from build123d import *

# Parameters (mm, degrees)
F1_DEPTH        = 5
F2_DEPTH        = 2.5
F3_R            = 8.24999
F4_R            = 13.24999
F5_R            = 13.24999
F6_R            = 15.24999
F7_DEPTH        = 4
F8_DEPTH        = 4
F9_R            = 4.99999
F11_D           = 3.1
F11_CSINK_D     = 6.1
F11_CSINK_ANGLE = 90
F13_D           = 3.1
F13_CSINK_D     = 6.1
F13_CSINK_ANGLE = 90
F14_R           = 1


# Not quite as in the source:
# - a fillet or chamfer is up to 0.001 mm smaller than in the source, because OpenCascade refuses the exact size


with BuildPart() as f1:
    # F0 (on Front) → F1 (new body, symmetric)
    with BuildSketch(Plane.XZ):
        Polygon((-20.0976822525, 0), (-7.0976822525, 0), (-7.0976822525, 8.25), (-7.0976822525, 16.5), (9.4023177475, 16.5), (9.4023177475, 0), (22.4023177475, 0), (22.4023177475, 5), (16.4023177475, 5), (14.4023177475, 5), (14.4023177475, 21.5), (-12.0976822525, 21.5), (-12.0976822525, 5), (-14.0976822525, 5), (-20.0976822525, 5), align=None)
    extrude(amount=F1_DEPTH, both=True)

    # F0 (on Front) → F2 (join, symmetric)
    with BuildSketch(Plane.XZ):
        Polygon((-14.0976822525, 23.5), (-14.0976822525, 5), (-12.0976822525, 5), (-12.0976822525, 21.5), (14.4023177475, 21.5), (14.4023177475, 5), (16.4023177475, 5), (16.4023177475, 23.5), align=None)
    extrude(amount=F2_DEPTH, both=True)

    # F3 (radius 8.25 in the source; OpenCascade refuses exactly that, so slightly less here)
    f3_edges = [f1.edges().sort_by_distance(p)[0] for p in [
        (-7.097682, 0, 16.5),
        (9.402318, 0, 16.5),
    ]]
    fillet(f3_edges, radius=F3_R)

    # F4 (radius 13.25 in the source; OpenCascade refuses exactly that, so slightly less here)
    f4_edges = [f1.edges().sort_by_distance(p)[0] for p in [
        (14.402318, -3.75, 21.5),
        (-12.097682, -3.75, 21.5),
    ]]
    fillet(f4_edges, radius=F4_R)

    # F5 (radius 13.25 in the source; OpenCascade refuses exactly that, so slightly less here)
    f5_edges = [f1.edges().sort_by_distance(p)[0] for p in [
        (14.402318, 3.75, 21.5),
        (-12.097682, 3.75, 21.5),
    ]]
    fillet(f5_edges, radius=F5_R)

    # F6 (radius 15.25 in the source; OpenCascade refuses exactly that, so slightly less here)
    f6_edges = [f1.edges().sort_by_distance(p)[0] for p in [
        (16.402318, 0, 23.5),
        (-14.097682, 0, 23.5),
    ]]
    fillet(f6_edges, radius=F6_R)

    # F7 (add): a face of the model
    f7_faces = [f1.faces().sort_by_distance(p)[0] for p in [
        (22.4023177475, 0, 2.5),
    ]]
    extrude(f7_faces, amount=F7_DEPTH)

    # F8 (add): a face of the model
    f8_faces = [f1.faces().sort_by_distance(p)[0] for p in [
        (-20.0976822525, 0, 2.5),
    ]]
    extrude(f8_faces, amount=F8_DEPTH)

    # F9 (radius 5 in the source; OpenCascade refuses exactly that, so slightly less here)
    f9_edges = [f1.edges().sort_by_distance(p)[0] for p in [
        (26.402318, -5, 2.5),
        (26.402318, 5, 2.5),
        (-24.097682, -5, 2.5),
        (-24.097682, 5, 2.5),
    ]]
    fillet(f9_edges, radius=F9_R)

    # F11 (through all)
    with Locations(Plane.XY.offset(5)):
        with Locations((-19.0976822525, 0)):
            CounterSinkHole(F11_D / 2, F11_CSINK_D / 2, counter_sink_angle=F11_CSINK_ANGLE)

    # F13 (through all)
    with Locations(Plane.XY.offset(5)):
        with Locations((21.4023177475, 0)):
            CounterSinkHole(F13_D / 2, F13_CSINK_D / 2, counter_sink_angle=F13_CSINK_ANGLE)

    # F14
    f14_edges = [f1.edges().sort_by_distance(p)[0] for p in [
        (-9.631064, -2.5, 19.033381),
        (-9.631064, 2.5, 19.033381),
        (17.902323, 5, 5),
        (-15.597687, 5, 5),
        (-12.097682, 5, 6.625005),
        (-8.21685, 5, 17.619168),
        (1.152318, 5, 21.5),
        (10.521486, 5, 17.619168),
        (14.402318, 5, 6.625005),
        (-22.633219, 3.535537, 5),
        (-24.097682, 0, 5),
        (-22.633219, -3.535537, 5),
        (-15.597687, -5, 5),
        (17.902323, -5, 5),
        (24.937855, -3.535537, 5),
        (26.402318, 0, 5),
        (24.937855, 3.535537, 5),
        (-14.097682, 2.5, 6.625005),
        (1.152318, 2.5, 23.5),
        (11.935699, 2.5, 19.033381),
        (16.402318, 2.5, 6.625005),
        (-14.097682, -2.5, 6.625005),
        (-12.097682, -5, 6.625005),
        (-8.21685, -5, 17.619168),
        (1.152318, -5, 21.5),
        (10.521486, -5, 17.619168),
        (14.402318, -5, 6.625005),
        (1.152318, -2.5, 23.5),
        (11.935699, -2.5, 19.033381),
        (16.402318, -2.5, 6.625005),
    ]]
    fillet(f14_edges, radius=F14_R)


solid = f1.part
Can you work these out from the model? Positions are in its coordinate system, mm. A direction names the side the tool comes from. Round coordinates to 2 decimals unless told otherwise and drop trailing zeros. Order: outer loops, then holes, each group sorted by start corner. A loop starts at its lowest first (then second) coordinate and runs counter-clockwise, first axis right, second up. Notation, with made-up numbers: (-22.5, 6) -> (20.5, 6) arc R15 cw to (20.5, 19) -> close; hole circle Ø7 at (71.25, 23). An arc over 180 degrees is marked (long way). Write each question's results on one line, items separated by ' | '. Start each with the question number.
Item 1: Thinking about a two-plate mould opening in X: for faces 4 (the cylindrical face through (17.458, 4.715, 4.699)), 5 (the flat face through (-14.098, 0, 7)), 6 (the cylindrical face through (16.102, 2.215, 6.602)), 7 (the flat face through (-7.098, 0, 4)), which applies, +X half, -X half, draft (parallel to the pull), parting line (faces both ways), or undercut?
Item 2: Which directions (+Z, -Z, +X, -X, +Y, -Y) give clear straight access to the entire face, cutting with the end or side of a thin tool? Please do faces 1 (the cylindrical face through (-11.8, -4.71, 6.57)), 2 (the cylindrical face through (-13.8, 2.21, 6.65)), 3 (the flat face through (14.402, 3, 7)).
Item 3: If we section it at B-B, the plane y = 1: State how many separate pieces and enclosed holes the cut face has, then the cut area to 3 significant figures.
Item 4: If we section it at A-A, the plane z = 7.75: Write out the boundary of the cut face in (x, y).
Item 5: Will these pins go through, and if not, where does the flat tip stop? pin 1 (2 mm diameter, centred on x = 15.5, z = 9.5, fed in from +Y); pin 2 (5 mm diameter, centred on y = -3.5, z = 14.5, fed in from +X); pin 3 (3 mm diameter, centred on y = 1, z = 13.5, fed in from +X).
Item 6: Please list where these lines run through material, in increasing order: L1, parallel to X at y = 0, z = 2.8; L2, parallel to X at y = 2.25, z = 10.25; L3, parallel to X at y = 1.25, z = 7.25.
Results:
1) face 4: draft | face 5: -X half | face 6: +X half | face 7: undercut
2) face 1: +Z, -X, -Y | face 2: +Z, -X, +Y | face 3: +Z, +X, +Y
3) separate pieces: 3 | enclosed holes: 0 | area: 444 mm2
4) outline: (-14.1, -1.5) arc R1 ccw to (-13.1, -2.5) -> (-12.1, -2.5) -> (-12.1, -4) arc R1 ccw to (-11.1, -5) -> (-7.1, -5) -> (-7.1, 5) -> (-11.1, 5) arc R1 ccw to (-12.1, 4) -> (-12.1, 2.5) -> (-13.1, 2.5) arc R1 ccw to (-14.1, 1.5) -> close; (9.4, -5) -> (13.4, -5) arc R1 ccw to (14.4, -4) -> (14.4, -2.5) -> (15.4, -2.5) arc R1 ccw to (16.4, -1.5) -> (16.4, 1.5) arc R1 ccw to (15.4, 2.5) -> (14.4, 2.5) -> (14.4, 4) arc R1 ccw to (13.4, 5) -> (9.4, 5) -> close
5) pin 1: stops at y = 2.5 | pin 2: stops at x = 15.7 | pin 3: stops at x = 15.93
6) L1: x = -24.1 to -20.65, -17.55 to -7.1, 9.4 to 19.85, 22.95 to 26.4 | L2: x = -13.62 to -6.85, 9.16 to 15.93 | L3: x = -14.1 to -7.1, 9.4 to 16.4
